Geometry: final body of the model. Coordinates: model frame, mm. Face numbers are marked on the shaded views. Give positions to 0.01 mm unless a question says otherwise; leave off trailing zeros. Loops run counter-clockwise (first coordinate to the right, second up) from the corner with the lowest first, then second, coordinate; pieces in that order, holes last. Notation, with made-up numbers: (49, 14.5) -> (55, 14.5) arc R20 cw to (55, 37.5) -> close; hole circle Ø2 at (45.5, -27). An arc over 180 degrees is marked (long way). Answer in a Markdown table with one row per item. Add a question column.
1) Section query C-C (z = 528.5). Return the cut outline in (x, y) (3 decimals), plus the area to 3 significant figures.
2) Section query B-B (x = 290). Return the cut outline in (y, z) (3 decimals), plus the area to 3 significant figures.
3) Section query A-A (z = -217.5). Return the cut outline in (x, y) (3 decimals).
4) First-contact query: P1, Ø11.5, axis at x = 538, z = -195, coming from the -Y side (3 decimals); P2, Ø2, axis at x = 501.5, y = -5, coming from the -Z side; P3, Ø5, axis at x = 274, y = -21, coming from the +Z side. Flat tips, straight axial feed; report the tip coordinate or a pass-through.
5) Draft query along Z for the marked faces 1 and 2. Return one class per face: +Z half, -Z half, draft (parallel to the pull), parting line (faces both ways), or undercut.
6) Line query: line 1 (X direction, y = -24, z = 863); line 2 (Y direction, x = 27, z = 372); line 3 (Y direction, x = 51, z = 203.5) (3 decimals). Output: solid intervals per line, ascending. Write a range as from..to.
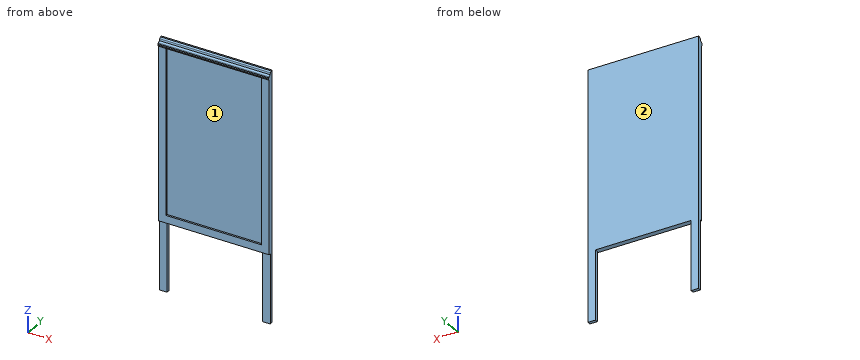
```python
from build123d import *

# Parameters (mm, degrees)
F0_W     = 558.8
F0_H     = 914.4
F1_DEPTH = 25.4
F2_W     = 482.6
F2_H     = 838.2
F3_DEPTH = 9.525
F4_W     = 38.1
F4_H     = 390.394981
F5_DEPTH = 15.875
F7_DEPTH = 558.801
F9_DEPTH = 558.8


with BuildPart() as f1:
    # F0 (on Front) → F1 (new body)
    with BuildSketch(Plane.XZ):
        with Locations((279.4, 457.2)):
            Rectangle(F0_W, F0_H)
    extrude(amount=F1_DEPTH)

    # F2 (on face) → F3 (cut)
    with BuildSketch(Plane.XZ.offset(25.4)):
        with Locations((279.4, 457.2)):
            Rectangle(F2_W, F2_H)
    extrude(amount=-F3_DEPTH, mode=Mode.SUBTRACT)

    # F4 (on face) → F5 (join, through all)
    with BuildSketch(Plane.XZ.offset(15.875)):
        with Locations((19.05, -157.09749)):
            Rectangle(F4_W, F4_H)
        with Locations((539.75, -157.09749)):
            Rectangle(F4_W, F4_H)
    extrude(amount=-F5_DEPTH)

    # F6 (on face) → F7 (cut, through all)
    with BuildSketch(Plane.YZ.offset(558.8)):
        Polygon((-14.501915, 908.10591), (-8.410952, 914.4), (-25.4, 914.4), (-25.4, 892.733455), (-17.402377, 899.984598), align=None)
    extrude(amount=-F7_DEPTH, mode=Mode.SUBTRACT)

    # F8 (on face) → F9 (join, through all)
    with BuildSketch(Plane.YZ.offset(558.8)):
        Polygon((-25.4, 876.3), (-25.4, 892.733455), (-28.536921, 889.689863), (-29.897201, 884.579603), (-28.536921, 880.158018), align=None)
    extrude(amount=-F9_DEPTH)


solid = f1.part
```
Evaluation:
| question | item | result |
|---|---|---|
| 1 | outline | (0, -25.4) -> (38.1, -25.4) -> (38.1, -15.875) -> (520.7, -15.875) -> (520.7, -25.4) -> (558.8, -25.4) -> (558.8, 0) -> (0, 0) -> close |
| 1 | area | 9,600 mm² |
| 2 | outline | (-29.897, 884.58) -> (-28.537, 880.158) -> (-25.4, 876.3) -> (-15.875, 876.3) -> (-15.875, 38.1) -> (-25.4, 38.1) -> (-25.4, 0) -> (0, 0) -> (0, 914.4) -> (-8.411, 914.4) -> (-14.502, 908.106) -> (-17.402, 899.985) -> (-25.4, 892.733) -> (-28.537, 889.69) -> close |
| 2 | area | 15,100 mm² |
| 3 | outline | (0, -15.875) -> (38.1, -15.875) -> (38.1, 0) -> (0, 0) -> close; (520.7, -15.875) -> (558.8, -15.875) -> (558.8, 0) -> (520.7, 0) -> close |
| 4 | P1 | y = -15.875 |
| 4 | P2 | z = 0 |
| 4 | P3 | z = 898.99 |
| 5 | face 1 | undercut |
| 5 | face 2 | draft |
| 6 | line 1 | 0..38.1, 520.7..558.8 |
| 6 | line 2 | -25.4..0 |
| 6 | line 3 | -15.875..0 |
